Part model, mm, in its own coordinate system. A direction names the side the tool comes from. Coordinates: 2 decimals unless noted, no trailing zeros. Loops run counter-clockwise (first coordinate to the right, second up) from the corner with the lowest first, then second, coordinate; pieces in that order, holes last. Notation, with made-up numbers: M 39,-39 L 94,-39 A24 ccw 94,-4 Z; hole C -9,62.5 d4. An arc over 180 degrees is marked long. Use a Markdown table: item, result. Add a question column.
1) Band-saw the part on A-A (y = -2.5). List the corners of the cut face in (x, z), plus the area to 3 significant figures.
2) Pin check, flat tips, straight feed: pin 1 Ø1.5 at (y, z) = (6, -3) entering from -X; pin 2 Ø3 at (y, z) = (-3.5, 2.5) entering from -X; pin 3 Ø1 at (x, z) = (2.5, -1) entering from +Y. Stop position of each tip, or through.
3) Tool access for faces 1 (the cylindrical face through (-2.579, 6.747, -1.978)), 2 (the flat face through (-1.725, 1.48, -3.045)): list every direction of +Z, -Z, +X, -X, +Y, -Y with a clear straight run to the whole face (end or side of a thin tool).
4) Pull direction Z, two halves, no side cores. Call faces 3 (the conical face through (2.376, 9.371, -0.985)), 4 (the cylindrical face through (-0.17, -5.3, -1.29)), 5 (the flat face through (1.8, 1.5, -3)): released by +Z, released by -Z, zero draft, split by the parting line, or undercut.
5) Band-saw the part on B-B (y = 4). List the corners of the cut face in (x, z), plus the area to 3 significant figures.
6) Wall check: probe 1 along X at (y, z) = (0.5, 0); probe 2 along X at (y, z) = (3.25, 1.25); probe 3 along Y at (x, z) = (0.25, 2). Give the ranges that are in metal, low to high. Write a range as from..to.
Solid Edge part; units mm, degrees
sketch "Sketch1" plane through (0, 0, 0) normal (0, 0, 1) x (1, 0, 0)
  arc A0 (0, 10.9) -> (1, 10.2583) centre (0, 9.8) cw
  line L0 (1, 10.2583) -> (1, 10.5)
  line L1 (1, 10.5) -> (2.0574, 10.5)
  line L2 (2.0574, 10.5) -> (2.3025, 10.3151)
  line L3 (2.3025, 10.3151) -> (3.25, 7)
  line L4 (3.25, 7) -> (3.25, 6.5)
  arc A1 (3.25, 6.5) -> (2.5, 4.5) centre (0.0009, 6.5778) cw
  arc A2 (2.5, 4.5) -> (3.3937, 3) centre (5.3226, 5.1655) ccw
  line L5 (3.3937, 3) -> (5.5, 1.7839)
  line L6 (5.5, 1.7839) -> (5.5, 1.2161)
  line L7 (5.5, 1.2161) -> (3.3937, 0)
  line L8 (3.3937, 0) -> (3.1027, -4.6517)
  line L9 (3.1027, -4.6517) -> (2.1996, -5.5)
  line L10 (2.1996, -5.5) -> (1.3, -5.5)
  line L11 (1.3, -5.5) -> (1.3, -5.1)
  arc A3 (1.3, -5.1) -> (1.7, -4.7) centre (1.3, -4.7) ccw
  line L12 (1.7, -4.7) -> (1.7, 9.55)
  line L13 (1.7, 9.55) -> (1.0067, 10.2433)
  arc A4 (1.0067, 10.2433) -> (0, 8.7) centre (0, 9.8) cw
  line L14 (0, 8.7) -> (0, 10.9)
revolve "RevolvedProtrusion1" add sketch "Sketch1" angle 360 about axis through (0, -5.5, 0) along (0, 1, 0)
sketch "Sketch2" plane through (0, 0, 0) normal (0, -1, 0) x (1, 0, 0)
  line L0 (-6, -6) -> (-6, 6)
  line L1 (-6, 6) -> (6, 6)
  line L2 (6, 6) -> (6, -6)
  line L3 (6, -6) -> (-6, -6)
  line L4 (-3.5, 2.0207) -> (0, 4.0415)
  line L5 (0, 4.0415) -> (3.5, 2.0207)
  line L6 (3.5, 2.0207) -> (3.5, -2.0207)
  line L7 (3.5, -2.0207) -> (0, -4.0415)
  line L8 (0, -4.0415) -> (-3.5, -2.0207)
  line L9 (-3.5, -2.0207) -> (-3.5, 2.0207)
extrude "Cutout1" cut sketch "Sketch2" against normal blind 3
properties part number "1/4-28 SAE-LT"
Entries:
| question | item | result |
|---|---|---|
| 1 | outline | C 0,0 d6.47; hole C 0,0 d3.4 |
| 1 | area | 23.8 mm2 |
| 2 | pin 1 | x = -2.29 |
| 2 | pin 2 | x = -3.02 |
| 2 | pin 3 | y = 10.4 |
| 3 | face 1 | +Y |
| 3 | face 2 | -Z, -X, +Y, -Y |
| 4 | face 3 | split by the parting line |
| 4 | face 4 | undercut |
| 4 | face 5 | released by -Z |
| 5 | outline | C 0,0 d5.33; hole C 0,0 d3.4 |
| 5 | area | 13.3 mm2 |
| 6 | probe 1 | -3.5..-1.7, 1.7..3.5 |
| 6 | probe 2 | -2.89..-1.15, 1.15..2.89 |
| 6 | probe 3 | -5.5..10.5 |
